Autodesk Inventor part; units mm, degrees
ref_plane "YZ Plane" through (0, 0, 0) normal (1, 0, 0) x (0, 1, 0)
ref_plane "XZ Plane" through (0, 0, 0) normal (0, 1, 0) x (-1, 0, 0)
ref_plane "XY Plane" through (0, 0, 0) normal (0, 0, 1) x (1, 0, 0)
ref_plane "Work Plane1" through (0, 0, 0) normal (0, 0, 1) x (1, 0, 0)
sketch "Sketch1" plane through (0, 0, 0) normal (0, 0, 1) x (1, 0, 0)
  line L0 (-1092.2, 304.8) -> (-1041.4, 304.8)
  line L1 (-50.8, -245.3386) -> (50.8, -304.8)
  line L2 (-1041.4, 304.8) -> (1524, 304.8)
  line L3 (-990.8062, 304.8) -> (-1092.2, 304.8)
  line L4 (-990.8062, 304.8) -> (-1092.2, 304.8)
  line L5 (-990.8062, 304.8) -> (-1092.2, 304.8)
  line L6 (50.8, -304.8) -> (-227.6342, -141.8464)
  line L7 (-227.6342, -141.8464) -> (-990.8062, 304.8)
  line L8 (-990.8062, 304.8) -> (-1092.2, 304.8)
  line L9 (-1092.2, 304.8) -> (-50.5938, -304.8)
  line L10 (50.8, -304.8) -> (-50.5938, -304.8)
  point P0 (-905.0447, 254.6081)
  point P1 (-930.9134, 210.407)
  point P2 (-162.6995, -179.8494)
extrude "Extrusion1" add sketch "Sketch1" against normal blind 50.8
properties part number "2x4x(24x43)"
Geometry check sheet. Reference: the model listing, model coordinates, mm. Coordinates: 2 decimals unless noted, no trailing zeros. Order: outer loops, then holes, each group sorted by start corner. A loop starts at its lowest first (then second) coordinate and runs counter-clockwise, first axis right, second up. Notation, with made-up numbers: M 54,23.25 L 75,23.25 A22 cw 75,32.25 Z; hole C -35,15.25 d4. An arc over 180 degrees is marked long. Use CSV: the item, a comma, the result in double quotes.
Item 1: Cross-section at B-B on x = -1007.5. Record the cut outline in (y, z).
Returned:
outline,"M 255.23,-50.8 L 304.8,-50.8 L 304.8,0 L 255.23,0 Z"
Item 2: Cross-section at A-A on z = -16. Record the cut outline in (x, y).
Returned:
outline,"M -1092.2,304.8 L -50.59,-304.8 L 50.8,-304.8 L -990.81,304.8 Z"
Item 3: Gauge pin test, flat ends, axial feed: pin 1 Ø5 at (y, z) = (154, -8.5) entering from +X; pin 2 Ø8 at (y, z) = (138.5, -32) entering from +X; pin 3 Ø3 at (y, z) = (-241, -44) entering from -X. Record the tip position at first contact, or that the pin passes through.
Returned:
pin 1,"stops at x = -728.87"
pin 2,"stops at x = -699.82"
pin 3,"stops at x = -162.17"
Item 4: Thickness scan on line 1 along X through (y, z) = (-134, -47); line 2 along X through (y, z) = (14, -8.5); line 3 along Y through (x, z) = (-786, -8). Record the ranges inside material, lowest first.
Returned:
line 1,"x = -342.43 to -241.04"
line 2,"x = -595.32 to -493.92"
line 3,"y = 125.6 to 184.94"
Item 5: Cross-section at C-C on y = -161. Record the cut outline in (x, z), then the cut area to 3 significant figures.
Returned:
outline,"M -296.3,-50.8 L -194.91,-50.8 L -194.91,0 L -296.3,0 Z"
area,"5,150 mm2"
